from build123d import *

# Parameters (mm, degrees)
SKETCH_R  = 1.5
PAD_DEPTH = 1.6


with BuildPart() as part:
    # Sketch → Pad (new body)
    with BuildSketch(Plane.XY):
        with BuildLine():
            ThreePointArc((59.5, 0), (43, 6), (26.5, 0))
            Line((26.5, 0), (26.5, 53))
            ThreePointArc((26.5, 53), (43, 47), (59.5, 53))
            ThreePointArc((66.5, 53), (63, 54.262411), (59.5, 53))
            ThreePointArc((66.5, 53), (76.280312, 47.553998), (87.365852, 45.996999))
            ThreePointArc((90.084619, 41.47693), (90.070775, 44.54629), (87.365852, 45.996999))
            ThreePointArc((90.084619, 41.47693), (86, 26.500006), (90.084613, 11.523081))
            ThreePointArc((87.365857, 7.003001), (90.070792, 8.45371), (90.084613, 11.523081))
            ThreePointArc((87.365857, 7.003001), (76.280314, 5.446003), (66.5, 0))
            ThreePointArc((59.5, 0), (63, -1.262442), (66.5, 0))
        make_face()
        with Locations((87.5, 43)):
            Circle(SKETCH_R, mode=Mode.SUBTRACT)
        with Locations((87.5, 10)):
            Circle(SKETCH_R, mode=Mode.SUBTRACT)
    extrude(amount=PAD_DEPTH)


solid = part.part
Design review of the part built by this model. Coordinates are the model's own, in mm. Round coordinates to 2 decimals unless told otherwise and drop trailing zeros. Write each loop counter-clockwise with the first axis right and the second up, starting at its lowest first coordinate (ties: lowest second). Pieces come first, ordered by that corner, then holes.
Item 1: For pin 1 Ø2.5 at (x, y) = (87.5, 10) entering from +Z, flat-tipped, find the tip position at first contact; note if it passes through.
Item 2: Draft analysis for pull direction Y (two halves, no side actions). For faces 1 (the cylindrical face through (89, 10, 1)), 2 (the cylindrical face through (43, 47, 1)), 3 (the cylindrical face through (62.947, -1.262, 0.789)), 4 (the flat face through (59, 27, 1.6)), state which applies: released by +Y, released by -Y, zero draft, split by the parting line, or undercut.
Item 3: Consider section C-C on y = 50. Give the boundary of the cut face in (x, z), and give its area (3 significant figures).
Item 4: Consider section B-B on z = 1.35. Give the boundary of the cut face in (x, y) (1 decimal).
Item 5: Consider section A-A on y = 43. Give the boundary of the cut face in (x, z), and give its area (3 significant figures).
Item 6: Consider section D-D on y = 33.5. Give the boundary of the cut face in (x, z).
Item 7: Wall thickness on L1, parallel to Y at x = 85.5, z = 0.8; L2, parallel to X at y = 26.5, z = 0.75; L3, parallel to Y at x = 43.5, z = 1.1: over which ranges is each line inside the solid? List them lowest first.
Check values:
1. pin 1: passes through
2. face 1: undercut
2. face 2: released by +Y
2. face 3: released by -Y
2. face 4: zero draft
3. outline: (26.5, 0) - (30.95, 0) - (30.95, 1.6) - (26.5, 1.6) - close; (55.05, 0) - (70.83, 0) - (70.83, 1.6) - (55.05, 1.6) - close
3. area: 32.4 mm2
4. outline: (26.5, 0) arc R25.7 cw to (59.5, 0) arc R5.5 ccw to (66.5, 0) arc R30.5 cw to (87.4, 7) arc R3 ccw to (90.1, 11.5) arc R29.5 cw to (90.1, 41.5) arc R3 ccw to (87.4, 46) arc R30.5 cw to (66.5, 53) arc R5.5 ccw to (59.5, 53) arc R25.7 cw to (26.5, 53) - close; hole circle Ø3 at (87.5, 10); hole circle Ø3 at (87.5, 43)
5. outline: (26.5, 0) - (86, 0) - (86, 1.6) - (26.5, 1.6) - close; (89, 0) - (90.5, 0) - (90.5, 1.6) - (89, 1.6) - close
5. area: 97.6 mm2
6. outline: (26.5, 0) - (86.84, 0) - (86.84, 1.6) - (26.5, 1.6) - close
7. L1: y = 7.03 to 45.97
7. L2: x = 26.5 to 86
7. L3: y = 6 to 47
